CAD build for the part. Positions are in the model's coordinates, mm. Face numbers are marked on the shaded views. Give positions to 0.01 mm unless a question says otherwise; leave off trailing zeros. Order: outer loops, then holes, each group sorted by start corner. A loop starts at its lowest first (then second) coordinate and runs counter-clockwise, first axis right, second up.
Item 1: Two-plate mould, pull along Y, no slides. Class the marked faces 1, 2, 3 and 4: released by +Y, released by -Y, zero draft, split by the parting line, or undercut.
Item 2: Band-saw the part on A-A on y = -1. Give the cut face in (x, z).
Item 3: Wall check: L1, parallel to Y at x = -99, z = 3; L2, parallel to Y at x = -84, z = 9; L3, parallel to X at y = -45, z = 0.75. Give the ranges that are in metal, low to high.
Item 4: Band-saw the part on B-B on z = 2.5. Give the cut face in (x, y), plus the area to 3 significant figures.
Item 5: Band-saw the part on C-C on x = -85.5. Give the cut face in (y, z), plus the area to 3 significant figures.
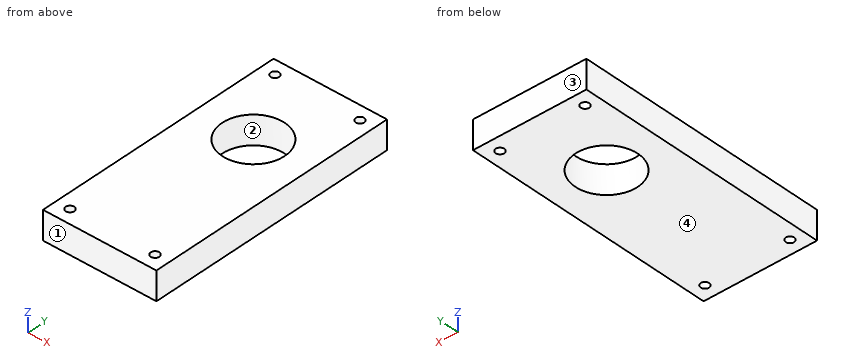
```python
from build123d import *
from build123d.topology import SkipClean

# Parameters (mm, degrees)
SKETCH1_R           = 1.5
BOSS_EXTRUDE1_DEPTH = 10


with BuildPart() as part:
    # Sketch1 → Boss-Extrude1 (new body)
    with BuildSketch(Plane.XY):
        with BuildLine():
            Line((-104.189078903, 39.114814762), (-104.189078903, -50.885185238))
            Line((-104.189078903, -50.885185238), (-84.189078903, -50.885185238))
            Line((-84.189078903, -50.885185238), (-84.189078903, -1.885185238))
            ThreePointArc((-84.189078903, -1.885185238), (-95.189078903, 9.114814762), (-84.189078903, 20.114814762))
            Line((-84.189078903, 20.114814762), (-84.189078903, 39.114814762))
            Line((-84.189078903, 39.114814762), (-104.189078903, 39.114814762))
        make_face()
        with Locations((-99.189078903, -45.885185238)):
            Circle(SKETCH1_R, mode=Mode.SUBTRACT)
        with Locations((-99.189078903, 34.114814762)):
            Circle(SKETCH1_R, mode=Mode.SUBTRACT)
    boss_extrude1 = extrude(amount=BOSS_EXTRUDE1_DEPTH)

    # Mirror1: Boss-Extrude1 across plane
    with SkipClean():  # the faces are left unmerged after this step: merging them gives an invalid solid
        add(boss_extrude1.mirror(Plane(origin=(-84.189078903, 0, 10), x_dir=(0, 0, 1), z_dir=(1, 0, 0))))


solid = part.part
```
The answers:
1. face 1: released by -Y
1. face 2: undercut
1. face 3: released by +Y
1. face 4: zero draft
2. outline: (-104.19, 0) - (-88.51, 0) - (-88.51, 10) - (-104.19, 10) - close; (-79.87, 0) - (-64.19, 0) - (-64.19, 10) - (-79.87, 10) - close
3. L1: y = -50.89 to -47.37, -44.4 to 32.63, 35.6 to 39.11
3. L2: y = -50.89 to -1.88, 20.11 to 39.11
3. L3: x = -104.19 to -100.4, -97.98 to -70.4, -67.98 to -64.19
4. outline: (-104.19, -50.89) - (-64.19, -50.89) - (-64.19, 39.11) - (-104.19, 39.11) - close; hole circle Ø3 at (-99.19, -45.89); hole circle Ø3 at (-99.19, 34.11); hole circle Ø22 at (-84.19, 9.11); hole circle Ø3 at (-69.19, -45.89); hole circle Ø3 at (-69.19, 34.11)
4. area: 3,190 mm2
5. outline: (-50.89, 0) - (-1.81, 0) - (-1.81, 10) - (-50.89, 10) - close; (20.04, 0) - (39.11, 0) - (39.11, 10) - (20.04, 10) - close
5. area: 682 mm2
